Can you work these out from the drawing? Everything is in mm from the part's minimum corner. Coordinates: 2 decimals unless noted, no trailing zeros. Write each loop counter-clockwise with the first axis right and the second up, starting at its lowest first coordinate (ties: lowest second). Pieces come first, ordered by that corner, then holes.
(1) Imagine slicing it at D-D, the plane z = 4. List the corners of the cut face in (x, y) for me, plus the area to 3 significant figures.
(2) Imagine slicing it at B-B, the plane x = 1.6. List the corners of the cut face in (y, z) for me, plus the area to 3 significant figures.
(3) Imagine slicing it at A-A, the plane z = 22.8. List the corners of the cut face in (x, y) for me.
(4) Please list where these lines run through material, in increasing order: probe 1 along Z at (x, y) = (4.1, 4.75); probe 2 along Y at (x, z) = (2.9, 22.8); probe 3 along Y at (x, z) = (2.9, 4).
(5) Imagine slicing it at C-C, the plane y = 3.5. List the corners of the cut face in (x, z) for me.
(6) For pin 1 Ø1 at (x, y) = (4.5, 2) entering from +Z, with a flat end and sliding along its axis, tell me the tip position at first contact or that it passes through.
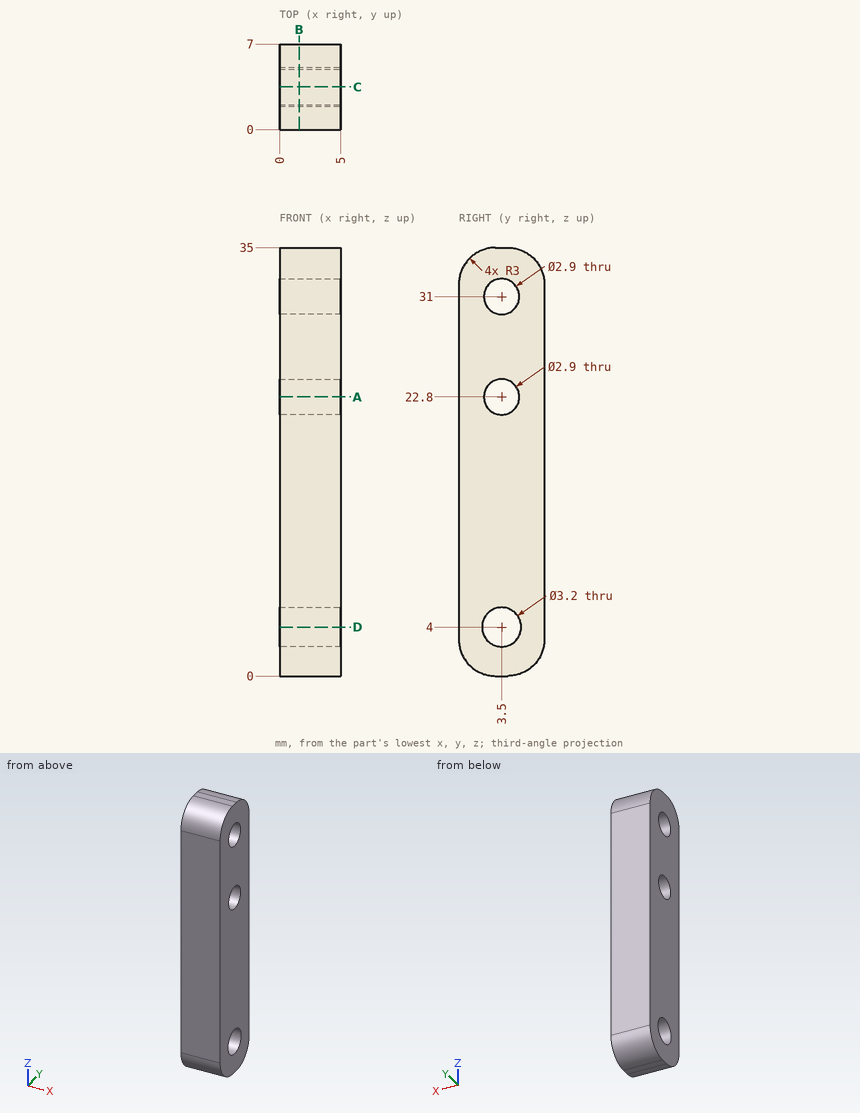
Recorded:
1. outline: (0, 0) - (5, 0) - (5, 1.9) - (0, 1.9) - close; (0, 5.1) - (5, 5.1) - (5, 7) - (0, 7) - close
1. area: 19.0 mm2
2. outline: (0, 3) arc R3 ccw to (3, 0) - (4, 0) arc R3 ccw to (7, 3) - (7, 32) arc R3 ccw to (4, 35) - (3, 35) arc R3 ccw to (0, 32) - close; hole circle Ø3.2 at (3.5, 4); hole circle Ø2.9 at (3.5, 22.8); hole circle Ø2.9 at (3.5, 31)
2. area: 216 mm2
3. outline: (0, 0) - (5, 0) - (5, 2.05) - (0, 2.05) - close; (0, 4.95) - (5, 4.95) - (5, 7) - (0, 7) - close
4. probe 1: z = 0.1 to 3, 5 to 22.07, 23.53 to 30.27, 31.73 to 34.9
4. probe 2: y = 0 to 2.05, 4.95 to 7
4. probe 3: y = 0 to 1.9, 5.1 to 7
5. outline: (0, 0) - (5, 0) - (5, 2.4) - (0, 2.4) - close; (0, 5.6) - (5, 5.6) - (5, 21.35) - (0, 21.35) - close; (0, 24.25) - (5, 24.25) - (5, 29.55) - (0, 29.55) - close; (0, 32.45) - (5, 32.45) - (5, 35) - (0, 35) - close
6. pin 1: stops at z = 34.96
